Geometry check sheet. Reference: the model listing, model coordinates, mm. A direction names the side the tool comes from. Coordinates: 2 decimals unless noted, no trailing zeros. Write each loop counter-clockwise with the first axis right and the second up, starting at its lowest first coordinate (ties: lowest second). Pieces come first, ordered by that corner, then holes. Notation, with made-up numbers: (-0.75, -7.75) -> (9.25, -7.75) arc R26 cw to (9.25, 22.25) -> close; hole circle Ø8 at (-2, -5.75). An arc over 180 degrees is marked (long way). Use a Markdown table: item, result.
Autodesk Inventor part; units mm, degrees
ref_plane "Work Plane11" through (7.5, 8.6447, 87.635) normal (0, 0.7071, -0.7071) x (-1, 0, 0)
ref_plane "Work Plane13" through (0, 0, 12.5) normal (0, 0, 1) x (1, 0, 0)
ref_plane "YZ Plane" through (0, 0, 0) normal (1, 0, 0) x (0, 1, 0)
sketch "Sketch1" plane through (0, 0, 0) normal (0, 1, 0) x (-1, 0, 0)
  arc A0 (-9.375, 11.7094) -> (9.375, 11.7094) centre (0, 0) ccw
  line L0 (-7.5, 15.6125) -> (-7.5, 22.9904)
  line L1 (7.5, 22.9904) -> (7.5, 15.6125)
  line L2 (7.5, 22.9904) -> (-7.5, 22.9904)
  arc A1 (7.5, 15.6125) -> (9.375, 11.7094) centre (12.5, 15.6125) ccw
  arc A2 (-9.375, 11.7094) -> (-7.5, 15.6125) centre (-12.5, 15.6125) ccw
  point P0 (7.5, 12.9904)
  point P1 (-7.5, 12.9904)
  point P2 (0, 12.9904)
  point P3 (0, 22.9904)
  dimension "d0" = 30
  dimension "d109" = 5
  dimension "d129" = 15
  dimension "d131" = 10
  dimension "d132" = 12.9904
extrude "Extrusion1" add sketch "Sketch1" against normal blind 12
sketch "Sketch22" plane through (-7.5, 0, 22.9904) normal (0, 0, 1) x (1, 0, 0)
  line L0 (0, 0) -> (0, -12)
  line L1 (15, -12) -> (0, -12)
  line L2 (0, 0) -> (15, 0)
  line L3 (15, 0) -> (15, -12)
  line L4 (15, -12) -> (0, -12)
  line L5 (0, -12) -> (0, 0)
  point P0 (7.5, 0)
sketch "Sketch23" plane through (0, 0, 0) normal (1, 0, 0) x (0, 1, 0)
  line L0 (0, 22.9904) -> (-12, 22.9904)
  line L1 (-6, 22.9904) -> (-6, 52.2797)
  line L2 (8.6447, 87.635) -> (43.4975, 122.4879)
  arc A0 (8.6447, 87.635) -> (-6, 52.2797) centre (44, 52.2797) ccw
  point P0 (0, 0)
  point P1 (-6, 72.9904)
  dimension "d110" = 50
  dimension "d111" = 70
  dimension "d112" = 135
  dimension "d113" = 50
sweep "Sweep2" add profiles "Sketch22" path "Sketch23" path curves L1 A0 L2
ref_plane "Work Plane11" through (7.5, 8.6447, 87.635) normal (0, 0.7071, -0.7071) x (-1, 0, 0)
sketch "Sketch24" plane through (7.5, 8.6447, 87.635) normal (0, 0.7071, -0.7071) x (-1, 0, 0)
  line L0 (0, 49.2893) -> (15, 49.2893)
  line L1 (0, 49.2893) -> (15, 49.2893)
  line L2 (0, 49.2893) -> (0, 53.2426)
  line L3 (15, 49.2893) -> (15, 53.2426)
  arc A0 (15, 53.2426) -> (0, 53.2426) centre (7.5, 61.2893) ccw
  point P0 (7.5, -68.08)
  point P1 (7.5, 49.2893)
  point P2 (7.5, 49.2893)
  dimension "d136" = 22
  dimension "d137" = 12
extrude "Extrusion17" add sketch "Sketch24" along normal mid plane 12
sketch "Sketch25" plane through (-7.5, 4.402, 91.8777) normal (0, -0.7071, 0.7071) x (1, 0, 0)
  circle A0 centre (7.5, 61.2893) radius 2.5
  arc A1 (15, 53.2426) -> (0, 53.2426) centre (7.5, 61.2893) ccw
  point P0 (7.5, -68.08)
  dimension "d123" = 5
extrude "Extrusion18" cut sketch "Sketch25" along normal through all both and the other way through all
sketch "Sketch26" plane through (0, -12, 0) normal (0, -1, 0) x (1, 0, 0)
  circle A0 centre (0, 0) radius 12.6
  dimension "d133" = 25.2
extrude "Extrusion19" cut sketch "Sketch26" against normal through all
sketch "Sketch28" plane through (7.5, 12.8873, 83.3924) normal (0, 0.7071, -0.7071) x (-1, 0, 0)
  circle A0 centre (7.5, 61.2893) radius 2.5
  circle A1 centre (7.5, 61.2893) radius 8.1
  point P0 (7.5, -68.08)
  dimension "d141" = 16.2
extrude "Extrusion21" cut sketch "Sketch28" against normal blind 5
mirror "Mirror3" about plane through (7.5, 8.6447, 87.635) normal (0, 0.7071, -0.7071) of "Extrusion21"
ref_plane "Work Plane13" through (0, 0, 12.5) normal (0, 0, 1) x (1, 0, 0)
properties part number "proximal_link_1"
Item 1: Section check D-D on z = 46. Record the boundary of the cut face in (x, y), then the cut area to 3 significant figures.
Answer block:
| item | result |
|---|---|
| outline | (-7.5, -12) -> (7.5, -12) -> (7.5, 0) -> (-7.5, 0) -> close |
| area | 180 mm^2 |
Item 2: Section check C-C on y = 33. Record the boundary of the cut face in (x, z).
Answer block:
| item | result |
|---|---|
| outline | (-7.5, 103.51) -> (7.5, 103.51) -> (7.5, 120.48) -> (-7.5, 120.48) -> close |
Item 3: Mould release check, pull along Y, two halves, no side actions. Record for faces 3 (the flat face through (0.105, 30.558, 101.063)), 4 (the flat face through (0, -12, 27)), 5 (the cylindrical face through (-7.48, 51.68, 135.67)): +Y half, -Y half, draft (parallel to the pull), parting line (faces both ways), or undercut.
Answer block:
| item | result |
|---|---|
| face 3 | +Y half |
| face 4 | -Y half |
| face 5 | undercut |
Item 4: Section check A-A on z = 0. Record the boundary of the cut face in (x, y).
Answer block:
| item | result |
|---|---|
| outline | (-15, -12) -> (-12.6, -12) -> (-12.6, 0) -> (-15, 0) -> close; (12.6, -12) -> (15, -12) -> (15, 0) -> (12.6, 0) -> close |
Item 5: Depth check by flat-ended pin: P1, Ø6, axis at x = -6.5, z = 104.5, coming from the +Y side; P2, Ø8, axis at x = 6, z = 96, coming from the +Y side; P3, Ø3, axis at x = -8, z = 123, coming from the +Y side (3 decimals); P4, Ø1, axis at x = 8.5, z = 101.5, coming from the -Y side. Enter the tip coordinate at first touch or a pass-through.
Answer block:
| item | result |
|---|---|
| P1 | stops at y = 36.99 |
| P2 | stops at y = 29.49 |
| P3 | stops at y = 53.995 |
| P4 | passes through |
Item 6: Section check B-B on x = 0. Count the separate pieces of the cut face and the enclosed holes in it, then the cut area to 3 significant figures.
Answer block:
| item | result |
|---|---|
| separate pieces | 3 |
| enclosed holes | 0 |
| area | 1,670 mm^2 |
Item 7: Thickness scan on L1, parallel to Y at x = -2.5, z = 40; L2, parallel to Z at x = 0, y = -5.75; L3, parallel to Z at x = 0, y = -4.5. Record the ranges inside material, lowest first. Write a range as [from, to].
Answer block:
| item | result |
|---|---|
| L1 | y = [-12, 0] |
| L2 | z = [-15, -12.6], [12.6, 77.99] |
| L3 | z = [-15, -12.6], [12.6, 80.28] |
Item 8: Tool access check on faces 1 (the cylindrical face through (0.11, -7.62, 73.99)), 2 (the flat face through (0, 0, 27)). Record the directions out of +Z, -Z, +X, -X, +Y, -Y that give a thin tool (end or side, any length) a straight path to the whole face; none if there is none.
Answer block:
| item | result |
|---|---|
| face 1 | +Z, +X, -X, -Y |
| face 2 | -Z, +X, -X, +Y |
